Could you check a few things on this drawing? It's one solid part, dimensions in mm from its lowest x, y, z. A direction names the side the tool comes from. Give positions to 0.01 mm unless a question says otherwise; leave off trailing zeros. Order: outer loops, then holes, each group sorted by start corner. A loop starts at its lowest first (then second) coordinate and runs counter-clockwise, first axis right, second up. Notation, with made-up numbers: (0.25, 46.5) - (54.25, 46.5) arc R22 cw to (54.25, 56.5) - close; hole circle Ø4 at (-17, -28.5). An arc over 180 degrees is marked (long way). Put each result on its own line as item: value.
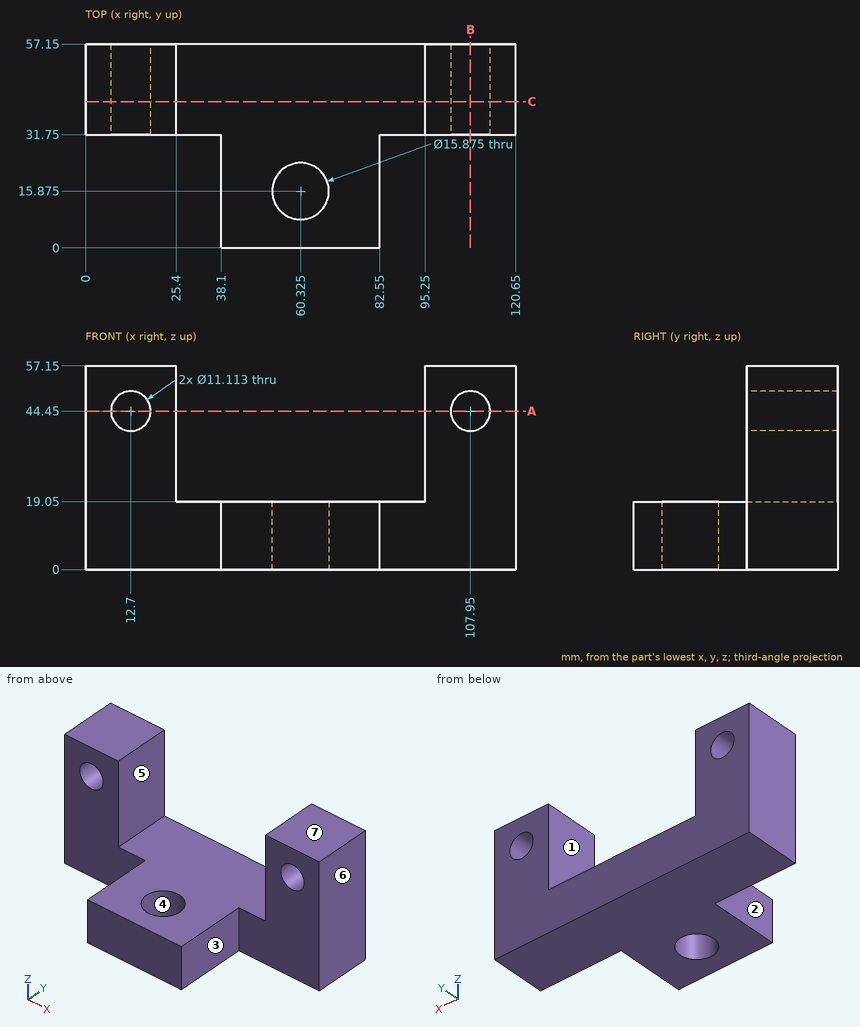
1) If I drill on line 1 (X direction, y = 42, z = 44); line 2 (Z direction, x = 107.95, y = 39.5); line 3 (X direction, y = 41, z = 36), over which ranges is the centre line in solid material (lowest first)? Write a range as [from, to].
Filled in:
line 1: x = [0, 7.16], [18.24, 25.4], [95.25, 102.41], [113.49, 120.65]
line 2: z = [0, 38.89], [50.01, 57.15]
line 3: x = [0, 25.4], [95.25, 120.65]
2) Suppose I cut it at B-B, the plane x = 107.95. List the corners of the cut face in (y, z) for me.
Filled in:
outline: (31.75, 0) - (57.15, 0) - (57.15, 38.89) - (31.75, 38.89) - close; (31.75, 50.01) - (57.15, 50.01) - (57.15, 57.15) - (31.75, 57.15) - close
3) I'm going to push flat-ended pins straight in: pin 1 (6 mm diameter, centred on y = 27.5, z = 38, fed in from +X); pin 2 (15 mm diameter, centred on y = 11.5, z = 13, fed in from -X); pin 3 (3 mm diameter, centred on x = 15.5, z = 33, fed in from -Y); pin 4 (9.5 mm diameter, centred on y = 12, z = 11, fed in from +X). Where does each tip first touch, or does it pass through?
Filled in:
pin 1: passes through
pin 2: stops at x = 38.1
pin 3: stops at y = 31.75
pin 4: stops at x = 82.55
4) Which directions (+Z, -Z, +X, -X, +Y, -Y) give clear straight access to the entire face, cutting with the end or side of a thin tool? Please do the marked faces 1, 2 and 3.
Filled in:
face 1: +Z, +Y, -Y
face 2: +Z, -Z, -X, -Y
face 3: +Z, -Z, +X, -Y
5) We'd pull the mould along X, two halves only. Please class the marked faces 4, 5, 6 and 7: pulls with the +X half, pulls with the -X half, needs draft (parallel to the pull), parting line crosses it, or undercut.
Filled in:
face 4: undercut
face 5: undercut
face 6: pulls with the +X half
face 7: needs draft
6) Suppose I cut it at C-C, the plane y = 41. List the corners of the cut face in (x, z) for me, and give its area (3 significant figures).
Filled in:
outline: (0, 0) - (120.65, 0) - (120.65, 57.15) - (95.25, 57.15) - (95.25, 19.05) - (25.4, 19.05) - (25.4, 57.15) - (0, 57.15) - close; hole circle Ø11.11 at (12.7, 44.45); hole circle Ø11.11 at (107.95, 44.45)
area: 4,040 mm^2
7) Suppose I cut it at A-A, the plane z = 44.45. List the corners of the cut face in (x, y) for me.
Filled in:
outline: (0, 31.75) - (7.14, 31.75) - (7.14, 57.15) - (0, 57.15) - close; (18.26, 31.75) - (25.4, 31.75) - (25.4, 57.15) - (18.26, 57.15) - close; (95.25, 31.75) - (102.39, 31.75) - (102.39, 57.15) - (95.25, 57.15) - close; (113.51, 31.75) - (120.65, 31.75) - (120.65, 57.15) - (113.51, 57.15) - close
